Design review of the part built by this model. Coordinates are the model's own, in mm. A direction names the side the tool comes from. Coordinates: 2 decimals unless noted, no trailing zeros. Write each loop counter-clockwise with the first axis right and the second up, starting at its lowest first coordinate (ties: lowest second). Pieces come first, ordered by that corner, then holes. Notation, with made-up numbers: M -19.5,10.5 L 13.5,10.5 A14 cw 13.5,24.5 Z; hole C -38.5,-6.75 d9. An arc over 180 degrees is marked long. Return JSON: item names as keys, results as strings. Group by question number.
```python
from build123d import *

# Parameters (mm, degrees)
HOLE_WIZARD_M4_1_D       = 3.3
SKETCH_4_R               = 3.25
CUT_EXTRUDE_1_DEPTH      = 3
SKETCH_5_R               = 1.75
CUT_EXTRUDE_2_DEPTH      = 49.744230428
PATTERN_CIRCULAR_1_COUNT = 4
CHAMFER_1_SIZE           = 0.5


with BuildPart() as part:
    # 草圖1 → 旋轉1 (revolve)
    with BuildSketch(Plane(origin=(0, 0, 0), x_dir=(0, 0, -1), z_dir=(1, 0, 0)), mode=Mode.PRIVATE) as revolve_1_sk:
        Polygon((0, 25.5), (0, 34), (7, 34), (7, 27), (11, 27), (11, 25.5), align=None)
    revolve(revolve_1_sk.sketch.rotate(Axis((0, 0, 0), (0, 0, -1)), 90), axis=Axis((0, 0, 0), (0, 0, -1)))

    # M4 螺紋孔1 (through all)
    with Locations(Plane.XY):
        with Locations((21.213203436, 21.213203436), (-21.213203436, -21.213203436)):
            Hole(HOLE_WIZARD_M4_1_D / 2)

    # 草圖4 → 伸長1 (cut)
    with BuildSketch(Plane.XY):
        with Locations((0, 30)):
            Circle(SKETCH_4_R)
    cut_extrude_1 = extrude(amount=-CUT_EXTRUDE_1_DEPTH, mode=Mode.SUBTRACT)

    # 草圖5 → 伸長2 (cut, through all)
    with BuildSketch(Plane.XY.offset(-3)):
        with Locations((0, 30)):
            Circle(SKETCH_5_R)
    cut_extrude_2 = extrude(amount=-CUT_EXTRUDE_2_DEPTH, mode=Mode.SUBTRACT)

    # 環狀複製排列1: 伸長1, 伸長2 ×4 about axis
    pattern_circular_1_axis = Axis((0, 0, 0), (0, 0, 1))
    add([cut_extrude_1.rotate(pattern_circular_1_axis, i * 360 / PATTERN_CIRCULAR_1_COUNT) for i in range(1, PATTERN_CIRCULAR_1_COUNT)], mode=Mode.SUBTRACT)
    add([cut_extrude_2.rotate(pattern_circular_1_axis, i * 360 / PATTERN_CIRCULAR_1_COUNT) for i in range(1, PATTERN_CIRCULAR_1_COUNT)], mode=Mode.SUBTRACT)

    # 導角1
    chamfer_1_edges = [part.edges().sort_by_distance(p)[0] for p in [
        (-34, 0, 0),
        (-25.5, 0, 0),
        (-27, 0, -11),
    ]]
    chamfer(chamfer_1_edges, length=CHAMFER_1_SIZE)


solid = part.part
```
Item 1: Add section C-C (z = -5). Write out the cut boundary in (x, y), plus the area to 3 significant figures.
Item 2: Add section A-A (y = 0). Count the separate pieces of the cut face and the enclosed holes in it, plus the area to 4 significant figures.
Item 3: Add section D-D (z = -9). Write out the cut boundary in (x, y).
Item 4: Machinability: for faces 1 (the flat face through (-14, -22, -11)), 2 (the flat face through (15, 23, -7)), 3 (the cylindrical face through (-0.705, 26.827, -1.479)), which of the approach directions +Z, -Z, +X, -X, +Y, -Y give a long, thin tool a straight path to every point of the face, cutting with its end or side? Answer none if there is none.
Item 5: The part is to be moulded in two halves that separate along Y. For faces 4 (the cylindrical face through (-5.85, 26.36, -8.77)), 5 (the flat face through (25, -8, 0)), 6 (the cylindrical face through (0.81, 28.45, -4.97)), say which applies: pulls with the +Y half, pulls with the -Y half, needs draft (parallel to the pull), parting line crosses it, or undercut.
Item 6: For line 1 (Y direction, x = 0, z = -1.6); line 2 (Y direction, x = 0, z = -4.75); line 3 (Y direction, x = 21, z = -1.25), list the stretches that pass through material, from the lowest coordinate up.
Item 7: For pin 1 (4 mm diameter, centred on x = 30, y = 0, fed in from -Z); pin 2 (2 mm diameter, centred on x = 0.5, y = 29, fed in from +Z); pin 3 (1.5 mm diameter, centred on y = 4, z = -4.5, fed in from +X), all flat-tipped, find the tip position at first contact; note any pin that passes through.
Geometry check:
{
 "1": {"outline": "C 0,0 d68; hole C -30,0 d3.5; hole C 0,0 d51; hole C -21.21,-21.21 d3.3; hole C 0,-30 d3.5; hole C 0,30 d3.5; hole C 21.21,21.21 d3.3; hole C 30,0 d3.5", "area": "1,530 mm^2"},
 "2": {"separate pieces": "4", "enclosed holes": "0", "area": "63.25 mm^2"},
 "3": {"outline": "C 0,0 d54; hole C 0,0 d51"},
 "4": {"face 1": "-Z, +X, -X, +Y, -Y", "face 2": "-Z", "face 3": "+Z"},
 "5": {"face 4": "parting line crosses it", "face 5": "needs draft", "face 6": "undercut"},
 "6": {"line 1": "-34 to -33.25, -26.75 to -25.5, 25.5 to 26.75, 33.25 to 34", "line 2": "-34 to -31.75, -28.25 to -25.5, 25.5 to 28.25, 31.75 to 34", "line 3": "-26.74 to -14.47, 14.47 to 19.58, 22.85 to 26.74"},
 "7": {"pin 1": "z = -7", "pin 2": "z = -3", "pin 3": "x = 33.84"}
}
